Part model, mm, in its own coordinate system. A direction names the side the tool comes from. Coordinates: 2 decimals unless noted, no trailing zeros. Loops run counter-clockwise (first coordinate to the right, second up) from the corner with the lowest first, then second, coordinate; pieces in that order, holes last. Notation, with made-up numbers: M 86.25,1 L 100.25,1 A17 cw 100.25,13 Z; hole C 42.25,78.25 d11. An arc over 180 degrees is marked long. Use a Markdown table: item, result. Add a question column.
1) Band-saw the part on B-B (z = -1). State how many separate pieces and enclosed holes the cut face has, plus the area to 3 significant figures.
2) Tool access for faces 1 (the flat face through (-9, 125, 1.588)), 2 (the cylindrical face through (-29.4, 98.24, -0.04)): list every direction of +Z, -Z, +X, -X, +Y, -Y with a clear straight run to the whole face (end or side of a thin tool).
3) Band-saw the part on C-C (y = 13.5). List the corners of the cut face in (x, z) (3 decimals), plus the area to 3 significant figures.
4) Band-saw the part on A-A (x = -29). List the corners of the cut face in (y, z) (3 decimals).
5) Wall check: probe 1 along X at (y, z) = (37.5, -1.5); probe 2 along X at (y, z) = (114, 1.75); probe 3 along X at (y, z) = (92, 0). Give the ranges that are in metal, low to high. Write a range as from..to.
6) Pin check, flat tips, straight feed: pin 1 Ø6 at (x, y) = (-7.13, 102.01) entering from +Z; pin 2 Ø1.5 at (y, z) = (68.5, 1.5) entering from -X; pin 3 Ø5 at (x, y) = (46, 48) entering from +Z. Stop position of each tip, or through.
7) Pull direction Y, two halves, no side cores. Call faces 3 (the flat face through (55.549, 77, 0)), 4 (the cylindrical face through (49.813, 37.285, -0.044)), 5 (the flat face through (48, 44, 1.588)): released by +Y, released by -Y, zero draft, split by the parting line, or undercut.
Autodesk Inventor part; units mm, degrees
ref_plane "YZ Plane" through (0, 0, 0) normal (1, 0, 0) x (0, 1, 0)
ref_plane "XZ Plane" through (0, 0, 0) normal (0, 1, 0) x (-1, 0, 0)
ref_plane "XY Plane" through (0, 0, 0) normal (0, 0, 1) x (1, 0, 0)
sketch "Sketch1" plane through (0, 0, 0) normal (0, 0, 1) x (1, 0, 0)
  line L0 (-166.2465, 0) -> (95.1399, 0)
  line L1 (0, -97.3562) -> (0, 206.312)
  circle A0 centre (0, 0) radius 53.975 construction
  arc A1 (39.2886, 39.2886) -> (-55.3511, 4.8426) centre (0, 0) ccw
  line L2 (0, 0) -> (-102.554, 102.554) construction
  circle A2 centre (-50.2894, 50.2894) radius 11.1125
  circle A3 centre (-50.2894, 50.2894) radius 13.335 construction
  circle A4 centre (-50.2894, 50.2894) radius 39.37 construction
  circle A5 centre (-26.9875, 87.3943) radius 11.1125
  circle A6 centre (-26.9875, 87.3943) radius 10.16 construction
  circle A7 centre (-26.9875, 87.3943) radius 33.02 construction
  circle A8 centre (13.589, 89.6653) radius 14.2875
  circle A9 centre (13.589, 89.6653) radius 33.02 construction
  circle A10 centre (0, 0) radius 16.51 construction
  arc A11 (51.2312, 117.4993) -> (-105.7834, 37.5874) centre (-4.3145, 32.4274) ccw
  line L3 (-103.0059, 30.3685) -> (-71.575, -1.0624)
  line L4 (55.5488, 46.0238) -> (55.5488, 109.5238)
  arc A12 (55.5488, 109.5238) -> (51.2312, 117.4993) centre (46.0238, 109.5238) ccw
  arc A13 (-105.7834, 37.5874) -> (-103.0059, 30.3685) centre (-96.2707, 37.1036) ccw
  arc A14 (-71.575, -1.0624) -> (-55.3511, 4.8426) centre (-64.8398, 5.6727) ccw
  arc A15 (39.2886, 39.2886) -> (55.5488, 46.0238) centre (46.0238, 46.0238) ccw
  line L5 (0, 0) -> (46.0238, 46.0238) construction
  line L6 (0, 0) -> (-64.8398, 5.6727) construction
  circle A16 centre (-17.0625, 17.0625) radius 10.16 construction
  point P0 (55.5488, 1.2332)
  point P1 (-51.3036, -21.3339)
  point P2 (55.5488, 114.5184)
  point P3 (-105.911, 33.2736)
  dimension "d0" = 107.95
  dimension "d1" = 45
  dimension "d2" = 1.5875
  dimension "d3" = 22.225
  dimension "d4" = 26.67
  dimension "d5" = 78.74
  dimension "d6" = 22.225
  dimension "d7" = 20.32
  dimension "d8" = 66.04
  dimension "d9" = 43.815
  dimension "d10" = 66.04
  dimension "d11" = 28.575
  dimension "d12" = 33.02
  dimension "d13" = 40.64
  dimension "d43" = 9.525
  dimension "d44" = 9.525
  dimension "d56" = 45
  dimension "d57" = 130
  dimension "d58" = 101.6
  dimension "d59" = 44.45
  dimension "d60" = 63.5
  dimension "d61" = 20.32
  dimension "d63" = 46.99
  dimension "d64" = 26.9875
  dimension "d66" = 13.589
  dimension "d67" = 24.13
extrude "Base" add sketch "Sketch1" along normal mid plane 6.35 contours L3 A13 A11 L1 A8 A1 A14 L0 | L0 A14 L3 | L1 A8 A11 A12 L4 A15 A1
sketch "Sketch2" plane through (0, 0, 3.175) normal (0, 0, 1) x (1, 0, 0)
  circle A0 centre (13.589, 89.6653) radius 14.2875
  line L0 (-1.0525, 107.1143) -> (27.5194, 73.0637) construction
  line L1 (-7.133, 102.0122) -> (5.028, 112.2165) construction
  line L2 (21.439, 67.9615) -> (33.5999, 78.1658) construction
  line L3 (-138.0646, 0) -> (87.8177, 0)
  line L4 (0, -31.4282) -> (0, 161.6033)
  dimension "d20" = 44.45
  dimension "d21" = 15.875
  dimension "d73" = 40
hole "Encoder Mount Holes" at (-7.133, 102.0122, 3.175) at (5.028, 112.2165, 3.175) at (21.439, 67.9615, 3.175) at (33.5999, 78.1658, 3.175) direction (0, 0, -1) diameter 5.1054 end through all countersink diameter 9.779 countersink angle 82
sketch "Sketch4" plane through (0, 0, 3.175) normal (0, 0, 1) x (1, 0, 0)
  arc A0 (55.5488, 109.5238) -> (51.2312, 117.4993) centre (46.0238, 109.5238) ccw
  arc A1 (-105.7834, 37.5874) -> (-103.0059, 30.3685) centre (-96.2707, 37.1036) ccw
  arc A2 (-71.575, -1.0624) -> (-55.3511, 4.8426) centre (-64.8398, 5.6727) ccw
  arc A3 (39.2886, 39.2886) -> (55.5488, 46.0238) centre (46.0238, 46.0238) ccw
  arc A4 (39.2886, 39.2886) -> (-55.3511, 4.8426) centre (0, 0) ccw
  line L0 (0, 0) -> (-77.2258, 92.0341) construction
  line L1 (0, 0) -> (-11.1042, 126.9216) construction
  line L2 (-139.4188, 0) -> (90.6686, 0) construction
  line L3 (0, -34.2819) -> (0, 162.079) construction
  dimension "d69" = 5
  dimension "d70" = 40
  dimension "d71" = 120.142
  dimension "d72" = 127.4064
hole "Standoff Holes" at (-96.2707, 37.1036, 3.175) at (46.0238, 109.5238, 3.175) at (-11.1042, 126.9216, 3.175) at (-77.2258, 92.0341, 3.175) at (-64.8398, 5.6727, 3.175) at (46.0238, 46.0238, 3.175) direction (0, 0, -1) diameter 5.1054 end through all counterbore diameter 9.779 counterbore depth 1.5875
properties part number "back plate"
Entries:
| question | item | result |
|---|---|---|
| 1 | separate pieces | 1 |
| 1 | enclosed holes | 13 |
| 1 | area | 11,900 mm2 |
| 2 | face 1 | +Z |
| 2 | face 2 | +Z, -Z |
| 3 | outline | M -86.137,-3.175 L -53.898,-3.175 L -53.898,3.175 L -86.137,3.175 Z |
| 3 | area | 205 mm2 |
| 4 | outline | M 47.394,-3.175 L 76.466,-3.175 L 76.466,3.175 L 47.394,3.175 Z; M 98.323,-3.175 L 130.983,-3.175 L 130.983,3.175 L 98.323,3.175 Z |
| 5 | probe 1 | -105.79..-98.79, -93.75..-41, 41.77..50.27 |
| 5 | probe 2 | -64.88..1.84, 8.21..44.06, 47.99..54.43 |
| 5 | probe 3 | -86.62..-79.78, -74.67..-37.1, -16.87..-0.51, 27.68..55.55 |
| 6 | pin 1 | z = 1.01 |
| 6 | pin 2 | x = -99.58 |
| 6 | pin 3 | z = 1.59 |
| 7 | face 3 | zero draft |
| 7 | face 4 | released by -Y |
| 7 | face 5 | undercut |
